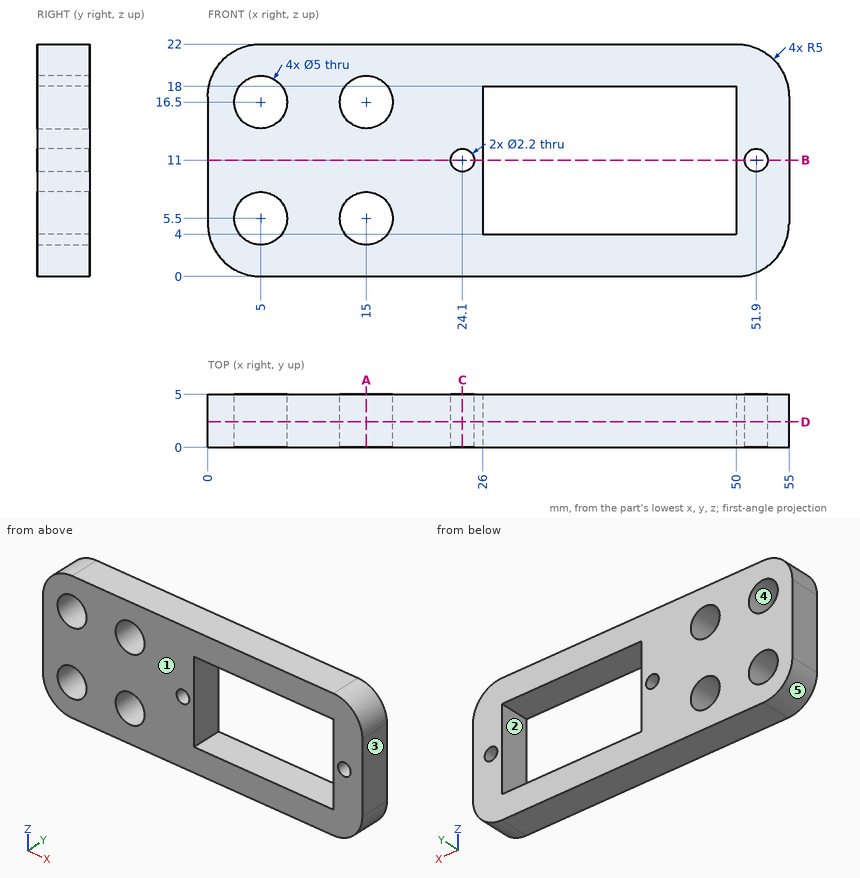
Can you work these out from the drawing? Everything is in mm from the part's minimum corner. A direction names the side the tool comes from. Round coordinates to 2 decimals unless told otherwise and drop trailing zeros. Write each loop counter-clockwise with the first axis right and the second up, starting at its lowest first coordinate (ties: lowest second). Pieces come first, ordered by that corner, then holes. Notation, with made-up numbers: (-19, 1.25) - (11, 1.25) arc R20 ccw to (11, 32.25) - close; hole circle Ø6 at (66.25, 73). An arc over 180 degrees is marked (long way). Write each question's results on one line, items separated by ' | '. Start each with the question number.
1) Which directions (+Z, -Z, +X, -X, +Y, -Y) give clear straight access to the entire face, cutting with the end or side of a thin tool? Please do the marked faces 1 and 2.
2) Suppose I cut it at C-C (x = 24.1). List the corners of the cut face in (y, z) for me.
3) Suppose I cut it at B-B (z = 11). List the corners of the cut face in (x, y) for me, and give its area (3 significant figures).
4) Suppose I cut it at A-A (x = 15). List the corners of the cut face in (y, z) for me, and give its area (3 significant figures).
5) Please list where these lines run through material, in increasing order: line 1 (X direction, y = 1.95, z = 11); line 2 (X direction, y = 2.05, z = 16.25); line 3 (X direction, y = 2.95, z = 18.5).
6) Suppose I cut it at D-D (y = 2.4). List the corners of the cut face in (x, z) for me.
7) For pin 1 Ø1.8 at (x, z) = (51.9, 11) entering from +Y, with a flat end and sliding along its axis, tell me the tip position at first contact or that it passes through.
8) We'd pull the mould along X, two halves only. Please class the marked faces 3, 4 and 5: released by +X, released by -X, zero draft, split by the parting line, or undercut.
Here are the results:
1) face 1: +Z, -Z, +X, -X, -Y | face 2: +Y, -Y
2) outline: (0, 0) - (5, 0) - (5, 9.9) - (0, 9.9) - close; (0, 12.1) - (5, 12.1) - (5, 22) - (0, 22) - close
3) outline: (0, 0) - (23, 0) - (23, 5) - (0, 5) - close; (25.2, 0) - (26, 0) - (26, 5) - (25.2, 5) - close; (50, 0) - (50.8, 0) - (50.8, 5) - (50, 5) - close; (53, 0) - (55, 0) - (55, 5) - (53, 5) - close | area: 133 mm2
4) outline: (0, 0) - (5, 0) - (5, 3) - (0, 3) - close; (0, 8) - (5, 8) - (5, 14) - (0, 14) - close; (0, 19) - (5, 19) - (5, 22) - (0, 22) - close | area: 60.0 mm2
5) line 1: x = 0 to 23, 25.2 to 26, 50 to 50.8, 53 to 55 | line 2: x = 0 to 2.51, 7.49 to 12.51, 17.49 to 26, 50 to 55 | line 3: x = 0.23 to 3.5, 6.5 to 13.5, 16.5 to 54.77
6) outline: (0, 5) arc R5 ccw to (5, 0) - (50, 0) arc R5 ccw to (55, 5) - (55, 17) arc R5 ccw to (50, 22) - (5, 22) arc R5 ccw to (0, 17) - close; hole circle Ø5 at (5, 5.5); hole circle Ø5 at (5, 16.5); hole circle Ø5 at (15, 5.5); hole circle Ø5 at (15, 16.5); hole circle Ø2.2 at (24.1, 11); hole (26, 4) - (50, 4) - (50, 18) - (26, 18) - close; hole circle Ø2.2 at (51.9, 11)
7) pin 1: passes through
8) face 3: released by +X | face 4: undercut | face 5: released by -X
